Geometry check sheet. Reference: the model listing, model coordinates, mm. Face numbers are marked on the shaded views. A direction names the side the tool comes from. Give positions to 0.01 mm unless a question says otherwise; leave off trailing zeros. Write each loop counter-clockwise with the first axis right and the second up, starting at its lowest first coordinate (ties: lowest second). Pieces come first, ordered by that corner, then holes. Notation, with made-up numbers: M -15,43.5 L 27,43.5 A35 ccw 27,80.5 Z; hole C 42.5,-35.5 d6. An arc over 180 degrees is marked long. One line per item, written item: value. Start each with the question number.
1. Gauge pin test, flat ends, axial feed: pin 1 (1 mm diameter, centred on x = 41.5, z = 6.5, fed in from -Y); pin 2 (1.5 mm diameter, centred on x = 36.5, y = -2, fed in from +Z) (3 decimals); pin 3 (1 mm diameter, centred on y = -5.5, z = 23, fed in from +X) (3 decimals). Record the tip position at first contact, or that the pin passes through.
2. Cross-section at B-B on y = -2.75. Record the cut outline in (x, z) (3 decimals).
3. Cross-section at A-A on x = 25. Record the cut outline in (y, z) (3 decimals).
4. Cross-section at D-D on x = 37.5. Record the cut outline in (y, z) (3 decimals), then the cut area to 3 significant figures.
5. Release check for a two-part mould opening along Z. For the marked faces 1, 2, 3 and 4 record: pulls with the +Z half, pulls with the -Z half, needs draft (parallel to the pull), parting line crosses it, or undercut.
6. Tool access check on the marked faces 5 and 6. Record the directions out of +Z, -Z, +X, -X, +Y, -Y that give a thin tool (end or side, any length) a straight path to the whole face; none if there is none.
7. Scan lines: line 1 (Z direction, x = 28.5, y = -2.5) (3 decimals); line 2 (X direction, y = -3.5, z = 10) (3 decimals); line 3 (Z direction, x = 26.5, y = 2.75) (3 decimals). Record each from-to range of solid material in increasing order.
Autodesk Inventor part; units mm, degrees
ref_plane "YZ Plane" through (0, 0, 0) normal (1, 0, 0) x (0, 1, 0)
ref_plane "XZ Plane" through (0, 0, 0) normal (0, 1, 0) x (-1, 0, 0)
ref_plane "XY Plane" through (0, 0, 0) normal (0, 0, 1) x (1, 0, 0)
sketch "Sketch1" plane through (0, 0, 0) normal (0, 1, 0) x (-1, 0, 0)
  line L0 (0, 0) -> (-50.8, 0)
  line L1 (-50.8, 0) -> (-50.8, 44.45)
  line L2 (-50.8, 44.45) -> (0, 44.45)
  line L3 (0, 44.45) -> (0, 0)
  dimension "d0" = 50.8
  dimension "d1" = 44.45
extrude "Extrusion1" add sketch "Sketch1" along normal blind 3.175
sketch "Sketch2" plane through (0, 0, 44.45) normal (0, -1, 0) x (1, 0, 0)
  line L0 (50.8, 0) -> (0, 0)
  line L1 (0, 0) -> (0, -44.45)
  line L2 (0, -44.45) -> (50.8, -44.45)
  line L3 (50.8, -44.45) -> (50.8, 0)
  line L4 (3.175, -3.175) -> (47.625, -3.175)
  line L5 (47.625, -3.175) -> (47.625, -41.275)
  line L6 (47.625, -41.275) -> (3.175, -41.275)
  line L7 (3.175, -41.275) -> (3.175, -3.175)
  dimension "d4" = 3.175
  dimension "d7" = 3.175
  dimension "d5" = 3.175
  dimension "d6" = 3.175
extrude "Extrusion2" add sketch "Sketch2" along normal blind 6.35
sketch "Sketch3" plane through (0, -6.35, 44.45) normal (0, 0, 1) x (1, 0, 0)
  line L0 (28.575, 0) -> (41.275, 0)
  line L1 (41.275, 0) -> (41.275, 6.35)
  line L2 (41.275, 6.35) -> (28.575, 6.35)
  line L3 (28.575, 6.35) -> (28.575, 0)
  line L4 (50.8, 0) -> (0, 0)
  line L5 (0, 9.525) -> (50.8, 9.525)
  line L6 (0, 9.525) -> (0, 0)
  dimension "d18" = 0
  dimension "d20" = 28.575
  dimension "d21" = 41.275
  dimension "d27" = 6.35
extrude "Extrusion3" cut sketch "Sketch3" against normal blind 3.175
sketch "Sketch4" plane through (50.8, 3.175, 44.45) normal (1, 0, 0) x (0, 0, -1)
  line L0 (0, 0) -> (0, -9.525)
  line L1 (44.45, -9.525) -> (0, -9.525)
  line L2 (12.7, -9.525) -> (25.4, -9.525)
  line L3 (25.4, -9.525) -> (25.4, -3.175)
  line L4 (25.4, -3.175) -> (12.7, -3.175)
  line L5 (12.7, -3.175) -> (12.7, -9.525)
  point P0 (44.45, -3.175)
  dimension "d22" = 6.35
  dimension "d23" = 12.7
  dimension "d24" = 25.4
extrude "Extrusion4" cut sketch "Sketch4" against normal blind 3.175
sketch "Sketch5" plane through (0, 3.175, 0) normal (0, 1, 0) x (1, 0, 0)
  line L0 (50.8, 0) -> (0, 0)
  line L1 (0, 0) -> (0, -44.45)
  line L2 (22.225, -9.525) -> (28.575, -9.525)
  line L3 (28.575, -9.525) -> (28.575, -15.875)
  line L4 (28.575, -15.875) -> (22.225, -15.875)
  line L5 (22.225, -15.875) -> (22.225, -9.525)
  dimension "d28" = 22.225
  dimension "d29" = 28.575
  dimension "d30" = 9.525
  dimension "d31" = 15.875
extrude "Extrusion5" cut sketch "Sketch5" against normal blind 3.175
sketch "Sketch6" plane through (0, 3.175, 0) normal (0, 1, 0) x (1, 0, 0)
  line L0 (50.8, 0) -> (0, 0)
  line L1 (0, 0) -> (0, -44.45)
  line L2 (0, -44.45) -> (50.8, -44.45)
  line L3 (6.35, 0) -> (7.9375, 0)
  line L4 (7.9375, 0) -> (7.9375, -44.45)
  line L5 (7.9375, -44.45) -> (6.35, -44.45)
  line L6 (6.35, -44.45) -> (6.35, 0)
  dimension "d34" = 1.5875
  dimension "d35" = 6.35
extrude "Extrusion6" cut sketch "Sketch6" against normal blind 1.5875 contours L4 L2 L6 L0
properties part number "Casing Top"
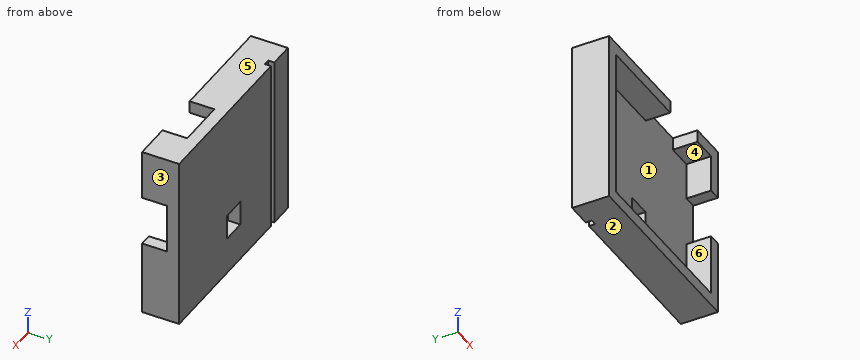
Report:
1. pin 1: stops at y = 0
1. pin 2: stops at z = 3.175
1. pin 3: stops at x = 3.175
2. outline: M 0,0 L 50.8,0 L 50.8,19.05 L 47.625,19.05 L 47.625,3.175 L 3.175,3.175 L 3.175,41.275 L 28.575,41.275 L 28.575,44.45 L 0,44.45 Z; M 41.275,41.275 L 47.625,41.275 L 47.625,31.75 L 50.8,31.75 L 50.8,44.45 L 41.275,44.45 Z
3. outline: M -6.35,0 L 3.175,0 L 3.175,9.525 L 0,9.525 L 0,3.175 L -6.35,3.175 Z; M -6.35,41.275 L 0,41.275 L 0,15.875 L 3.175,15.875 L 3.175,44.45 L -6.35,44.45 Z
4. outline: M -6.35,0 L 3.175,0 L 3.175,44.45 L 0,44.45 L 0,3.175 L -6.35,3.175 Z
4. area: 161 mm^2
5. face 1: undercut
5. face 2: pulls with the -Z half
5. face 3: needs draft
5. face 4: undercut
6. face 5: +Z, +X, -X, +Y, -Y
6. face 6: -Y
7. line 1: z = 0 to 3.175, 41.275 to 44.45
7. line 2: x = 0 to 3.175, 47.625 to 50.8
7. line 3: z = 0 to 9.525, 15.875 to 44.45
